The listing builds one solid part. Answer for the finished solid, in the listing's coordinates (mm). A direction names the side the tool comes from. Round coordinates to 2 decimals unless told otherwise and drop trailing zeros. Order: outer loops, then holes, each group sorted by start corner. A loop starts at its lowest first (then second) coordinate and runs counter-clockwise, first axis right, second up. Notation, with made-up numbers: (23.25, 66.5) - (67.25, 66.5) arc R19 ccw to (67.25, 82.5) - close; hole circle Ø9 at (48.25, 8.25). An arc over 180 degrees is marked (long way). One line per item, written item: value. Start each with the question number.
1. A tool of negligible diameter and unlimited length cuts with its end or side. For faces 1 (the flat face through (7, 0, 0.35)), 2 (the flat face through (4, -4, 0.7)), 3 (the flat face through (-5.54, -2.706, 0.368)), from which of +Z, -Z, +X, -X, +Y, -Y can it reach the whole face along a straight path? Write none if from no direction.
2. Straight lines are drawn through the part: line 1 (Y direction, x = 0, z = 0.35); line 2 (X direction, y = 0, z = 0.5); line 3 (X direction, y = 0, z = 0.45). For each, find the intervals that lie inside material, in ascending order.
3. For a pull along Y with two mould halves and no side action, classify faces 4 (the flat face through (-10.1, 1.1, 2)), 5 (the cylindrical face through (2.93, -13.18, 0.99)), 6 (the flat face through (5.54, 2.706, 0.173)) as released by +Y, released by -Y, zero draft, split by the parting line, or undercut.
4. Section A-A, the plane y = 11 is taken. Give the vertices of the cut face in (x, z), then the cut area to 3 significant figures.
5. Flat-ended cylindrical pins translate along their axes: P1, Ø5, axis at x = -3.5, y = -4, coming from the +Z side; P2, Ø6.5, axis at x = 5.5, y = 0, coming from the -Z side; P3, Ø8.5, axis at x = 0, y = 0, coming from the -Z side; P4, Ø1, axis at x = -2.5, z = 2, coming from the +Y side. Find the tip coordinate at first contact, or state that the pin passes through.
from build123d import *

# Parameters (mm, degrees)
F3_DEPTH = 0.35
F4_DEPTH = 5


with BuildPart() as f1:
    # F0 (on Front) → F1 (revolve)
    with BuildSketch(Plane.XZ):
        with BuildLine():
            add(Edge.make_bspline(
                [(-10, 2), (-9.8134251311, 1.2643112568), (-9.5979757607, 0.7219304822), (-8.6464062333, 0.7)],
                knots=[0, 0, 0, 0, 1.8767567997, 1.8767567997, 1.8767567997, 1.8767567997], degree=3))
            Line((-10, 2), (-13.5, 2))
            Line((-13.5, 2), (-13.5, 0))
            Line((-13.5, 0), (-4.7, 0))
            Line((-4.7, 0), (-4.7, 0.7))
            Line((-4.7, 0.7), (-8.6464062333, 0.7))
        make_face()
    revolve(axis=Axis((0, 0, 0.3460962325), (0, 0, -1)))

    # F2 (on Top) → F3 (cut)
    with BuildSketch(Plane.XY):
        with BuildLine():
            Line((9.4376522897, 1), (1.5316589494, 4.4600760879))
            Line((1.5316589494, 4.4600760879), (1.5316589494, -4.4600760879))
            Line((1.5316589494, -4.4600760879), (9.4376522897, -1))
            ThreePointArc((9.4376522897, -1), (10.0915766243, 0), (9.4376522897, 1))
        make_face()
    extrude(amount=F3_DEPTH, mode=Mode.SUBTRACT)

    # F2 (on Top) → F4 (cut)
    with BuildSketch(Plane.XY):
        with BuildLine():
            Line((-1.5316589494, -4.4600760879), (-1.5316589494, 4.4600760879))
            Line((-1.5316589494, 4.4600760879), (-9.4376522897, 1))
            ThreePointArc((-9.4376522897, 1), (-10.0915766243, 0), (-9.4376522897, -1))
            Line((-9.4376522897, -1), (-1.5316589494, -4.4600760879))
        make_face()
    extrude(amount=F4_DEPTH, mode=Mode.SUBTRACT)

    # F5 (on Front) → F6 (revolve, cut)
    with BuildSketch(Plane.XZ):
        Polygon((7.8459653944, 0.038968916), (9, 0), (13.550709933, 2), (13.3823033062, 2.4721443956), align=None)
    revolve(axis=Axis((11.2753549665, 0, 1), (0.9154864336, 0, 0.402348841)), mode=Mode.SUBTRACT)

    # F5 (on Front) → F7 (revolve, cut)
    with BuildSketch(Plane.XZ):
        Polygon((-13.3823033062, 2.4721443956), (-13.550709933, 2), (-9, 0), (-7.8459653944, 0.038968916), align=None)
    revolve(axis=Axis((-11.2753549665, 0, 1), (-0.9154864336, 0, 0.402348841)), mode=Mode.SUBTRACT)


solid = f1.part
Answer list:
1. face 1: -Z
1. face 2: +Z
1. face 3: +Z, -Z
2. line 1: y = -13.5 to -4.7, 4.7 to 13.5
2. line 2: x = -13.5 to -11.38, 4.7 to 8.89, 11.38 to 13.5
2. line 3: x = -13.5 to -11.27, 4.7 to 8.78, 11.27 to 13.5
3. face 4: zero draft
3. face 5: split by the parting line
3. face 6: undercut
4. outline: (-7.83, 0) - (7.83, 0) - (7.83, 2) - (-7.83, 2) - close
4. area: 31.3 mm²
5. P1: stops at z = 0.7
5. P2: stops at z = 0
5. P3: passes through
5. P4: stops at y = 13.35
